Part model, mm, in its own coordinate system. Round coordinates to 2 decimals unless told otherwise and drop trailing zeros. Write each loop counter-clockwise with the first axis right and the second up, starting at its lowest first coordinate (ties: lowest second). Pieces come first, ordered by that corner, then holes. Notation, with made-up numbers: M 16,69 L 70,69 A18 ccw 70,78 Z; hole C -35.75,78 d5. An arc over 180 degrees is marked long. Answer as a JSON object with one key per item and string values. Group by question number.
1. Band-saw the part on A-A, the plane z = 1.85. Count the separate pieces of the cut face and the enclosed holes in it, plus the area to 3 significant figures.
2. Drill centre lines: line 1 (Y direction, x = -4.5, z = 1.9); line 2 (Y direction, x = 28.5, z = 2.3); line 3 (X direction, y = -28.5, z = 2.1). Where is each one in solid material? Low to high. Write a range as from..to.
3. Drop flat-ended pins along their axis: pin 1 (1.5 mm diameter, centred on x = -17, z = 1.5, fed in from -Y); pin 2 (1.5 mm diameter, centred on y = -1, z = 1.5, fed in from +X); pin 3 (5 mm diameter, centred on x = 86.5, y = -41.5, fed in from -Z); pin 4 (1.5 mm diameter, centred on x = 3, z = 1.5, fed in from -Y). Give the stop position or say it passes through.
4. Band-saw the part on B-B, the plane x = 64.5. Write the cut outline in (y, z), plus the area to 3 significant figures.
5. Band-saw the part on C-C, the plane y = -21.5. Write the cut outline in (x, z).
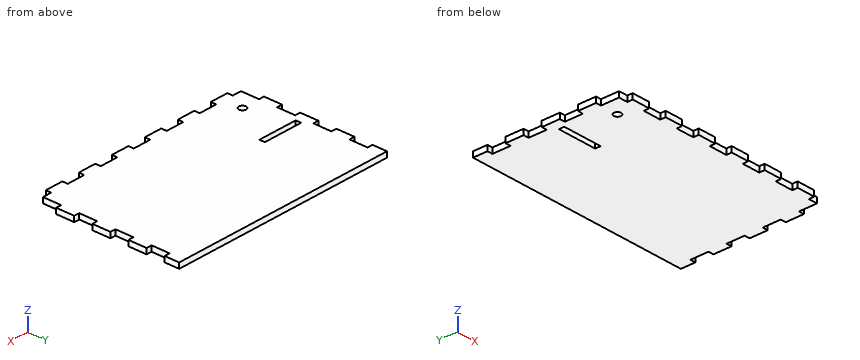
Autodesk Inventor part; units mm, degrees
ref_plane "YZ Plane" through (0, 0, 0) normal (1, 0, 0) x (0, 1, 0)
ref_plane "XZ Plane" through (0, 0, 0) normal (0, 1, 0) x (-1, 0, 0)
ref_plane "XY Plane" through (0, 0, 0) normal (0, 0, 1) x (1, 0, 0)
ref_plane "Work Plane2" through (0, 0, 0) normal (0, 0, 1) x (1, 0, 0)
sketch "Sketch2" plane through (0, 0, 0) normal (0, 0, 1) x (1, 0, 0)
  line L0 (-13, 0) -> (-13, 3)
  line L1 (-13, 3) -> (-10, 3)
  line L2 (103, 0) -> (103, 3)
  line L3 (100, 3) -> (103, 3)
  line L4 (103, 8) -> (-13, 8)
  line L5 (-10, 0) -> (-10, 3)
  line L6 (-10, 3) -> (0, 3)
  line L7 (100, 0) -> (100, 3)
  line L8 (90, 3) -> (100, 3)
  line L9 (90, 3) -> (0, 3)
  line L10 (0, 0) -> (90, 0)
  line L11 (0, 0) -> (0, 3)
  line L12 (90, 0) -> (90, 3)
  line L13 (90, 3) -> (90, 0)
  line L14 (0, 3) -> (0, 0)
  line L15 (45, 0) -> (45, -20) construction
  line L16 (-15.0005, 0) -> (-15.0005, -10)
  line L17 (-15.0005, -10) -> (-18.0005, -10)
  line L18 (-15.0005, -20) -> (-18.0005, -20)
  line L19 (-15.0005, -20) -> (-15.0005, -30)
  line L20 (-15.0005, -30) -> (-18.0005, -30)
  line L21 (-15.0005, -40) -> (-18.0005, -40)
  line L22 (-15.0005, -50) -> (-18.0005, -50)
  line L23 (-15.0005, -60) -> (-18.0005, -60)
  line L24 (-18.0005, -10) -> (-18.0005, -20)
  line L25 (-18.0005, -30) -> (-18.0005, -40)
  line L26 (-18.0005, -50) -> (-18.0005, -60)
  line L27 (-15.0005, -40) -> (-15.0005, -50)
  line L28 (90, -73) -> (90, -70)
  line L29 (80, -73) -> (70, -73)
  line L30 (60, -73) -> (50, -73)
  line L31 (45, -70) -> (45, -47.72) construction
  line L32 (80, -73) -> (80, -70)
  line L33 (70, -73) -> (70, -70)
  line L34 (60, -73) -> (60, -70)
  line L35 (90, -70) -> (80, -70)
  line L36 (80, -73) -> (70, -73)
  line L37 (70, -70) -> (60, -70)
  line L38 (-10, -73) -> (0, -73)
  line L39 (0, -73) -> (0, -70)
  line L40 (10, -73) -> (20, -73)
  line L41 (10, -73) -> (10, -70)
  line L42 (20, -73) -> (20, -70)
  line L43 (30, -73) -> (30, -70)
  line L44 (0, -70) -> (10, -70)
  line L45 (20, -70) -> (30, -70)
  line L46 (60, -73) -> (50, -73)
  line L47 (50, -73) -> (50, -70)
  line L48 (50, -70) -> (45, -70)
  line L49 (45, -70) -> (40, -70)
  line L50 (40, -70) -> (40, -73)
  line L51 (30, -73) -> (40, -73)
  line L52 (50, -73) -> (77.2719, -73)
  line L53 (60, -73) -> (50, -73)
  line L54 (45, -70) -> (40, -70)
  line L55 (40, -73) -> (30, -73)
  line L56 (30, -70) -> (20, -70)
  line L57 (10, -70) -> (0, -70)
  line L58 (20, -73) -> (10, -73)
  line L59 (0, -73) -> (12.7281, -73)
  line L60 (-18, 8) -> (-13, 8)
  line L61 (-15.0005, 0) -> (-18, 0)
  line L62 (-15.0005, -60) -> (-15.0005, -70)
  line L63 (-18, -50) -> (-18, -60)
  line L64 (-18, -30) -> (-18, -40)
  line L65 (-18, 8) -> (-18, 0)
  line L66 (-18, -10) -> (-18, -20)
  line L67 (105.0005, 0) -> (105.0005, -10)
  line L68 (108.0005, -10) -> (108.0005, -20)
  line L69 (105.0005, -10) -> (108.0005, -10)
  line L70 (105.0005, -20) -> (108.0005, -20)
  line L71 (105.0005, -20) -> (105.0005, -30)
  line L72 (105.0005, -30) -> (108.0005, -30)
  line L73 (108.0005, -30) -> (108.0005, -40)
  line L74 (105.0005, -40) -> (108.0005, -40)
  line L75 (105.0005, -40) -> (105.0005, -50)
  line L76 (105.0005, -50) -> (108.0005, -50)
  line L77 (108.0005, -50) -> (108.0005, -60)
  line L78 (105.0005, -60) -> (108.0005, -60)
  line L79 (108, 8) -> (103, 8)
  line L80 (105.0005, 0) -> (108, 0)
  line L81 (105.0005, -60) -> (105.0005, -70)
  line L82 (108, -50) -> (108, -60)
  line L83 (108, -30) -> (108, -40)
  line L84 (108, 8) -> (108, 0)
  line L85 (108, -10) -> (108, -20)
  line L86 (100, -73) -> (90, -73)
  line L87 (0, -73) -> (-10, -73)
  line L88 (-10, -73) -> (-10, -70)
  line L89 (-10, -70) -> (-15.0005, -70)
  line L90 (-13, -73) -> (-10, -73)
  line L91 (100, -73) -> (98, -73)
  line L92 (90, -70) -> (100, -70)
  line L93 (100, -70) -> (100, -73)
  line L94 (105.0005, -70) -> (100, -70)
  dimension "d39" = 10
  dimension "d42" = 10
extrude "Extrusion1" add sketch "Sketch2" along normal blind 3 contours L79 L84 L80 L67 L69 L68 L70 L71 L72 L73 L74 L75 L76 L77 L78 L81 L94 L92 L35 L32 L29 L33 L37 L34 L30 L47 L48 L49 L50 L51 L43 L45 L42 L40 L41 L44 L39 L38 L88 L89 L62 L23 L26 L22 L27 L21 L25 L20 L19 L18 L24 L17 L16 L61 L65 L60 L4 | L93 L86 L28 L92 | L12 L10 L11 L9
sketch "Sketch3" plane through (0, 0, 3) normal (0, 0, 1) x (1, 0, 0)
  line L0 (0, -70) -> (10, -70)
  line L1 (-15.0005, -40) -> (-15.0005, -50)
  line L2 (-9.2505, -64.25) -> (7.7495, -64.25)
  line L3 (7.7495, -64.25) -> (7.7495, -55.25)
  line L4 (7.7495, -55.25) -> (-9.2505, -55.25)
  line L5 (-9.2505, -55.25) -> (-9.2505, -64.25)
  line L6 (16.5, -70) -> (16.5, 3)
  line L7 (13.5, 3) -> (13.5, -70)
  circle A0 centre (-5.0005, -60) radius 2
  line L8 (-15.0005, -60) -> (-15.0005, -70)
  line L9 (-15.0005, -70) -> (-10, -70)
  point P0 (0, 0)
  dimension "d57" = 17
  dimension "d58" = 9
  dimension "d59" = 5.75
  dimension "d60" = 5.75
  dimension "d61" = 4
  dimension "d62" = 10
  dimension "d63" = 10
extrude "Extrusion2" cut sketch "Sketch3" against normal blind 10 contours A0
sketch "Sketch4" plane through (0, 0, 3) normal (0, 0, 1) x (1, 0, 0)
  line L0 (-12, -37) -> (10, -37)
  line L1 (10, -37) -> (10, -34)
  line L2 (10, -34) -> (-12, -34)
  line L3 (-12, -34) -> (-12, -37)
  line L4 (108, 8) -> (-18, 8)
  line L5 (-18, -30) -> (-18, -40)
  dimension "d51" = 22
  dimension "d52" = 3
  dimension "d53" = 45
  dimension "d54" = 6
extrude "Extrusion3" cut sketch "Sketch4" against normal blind 10
properties part number "back"
Worked answers:
{
 "1": {"separate pieces": "1", "enclosed holes": "2", "area": "9,690 mm^2"},
 "2": {"line 1": "y = -73..-61.94, -58.06..-37, -34..8", "line 2": "y = -70..8", "line 3": "x = -15..105"},
 "3": {"pin 1": "stops at y = -60", "pin 2": "stops at x = 105", "pin 3": "stops at z = 0", "pin 4": "stops at y = -70"},
 "4": {"outline": "M -70,0 L 8,0 L 8,3 L -70,3 Z", "area": "234 mm^2"},
 "5": {"outline": "M -15,0 L 105,0 L 105,3 L -15,3 Z"}
}
